Verification items for the finished model (mm, model axes). A direction names the side the tool comes from. Coordinates: 2 decimals unless noted, no trailing zeros. Order: outer loops, then holes, each group sorted by start corner. A loop starts at its lowest first (then second) coordinate and runs counter-clockwise, first axis right, second up. Notation, with made-up numbers: M 65,29 L 76,29 A34 ccw 76,66 Z; hole C 68,63.25 d2. An arc over 180 degrees is marked long. Write item = value, one per line.
```python
from build123d import *

# Parameters (mm, degrees)
F0_R     = 20
F1_DEPTH = 450
F2_R     = 35
F3_DEPTH = 24
F4_W     = 60
F4_H     = 45
F5_DEPTH = 25
F5_TAPER = -18.1


with BuildPart() as f1:
    # F0 (on Top) → F1 (new body)
    with BuildSketch(Plane.XY):
        Circle(F0_R)
    extrude(amount=F1_DEPTH)

    # F2 (on face) → F3 (join)
    with BuildSketch(Plane.XY.offset(450)):
        Circle(F2_R)
    extrude(amount=F3_DEPTH)

    # F4 (on Top) → F5 (join)
    with BuildSketch(Plane.XY):
        Rectangle(F4_W, F4_H)
    extrude(amount=-F5_DEPTH, taper=F5_TAPER)


solid = f1.part
```
Item 1: Gauge pin test, flat ends, axial feed: pin 1 (6 mm diameter, centred on y = 2, z = 206.5, fed in from -X); pin 2 (10 mm diameter, centred on x = -18.5, z = 53, fed in from +Y); pin 3 (10 mm diameter, centred on y = 22.5, z = 355.5, fed in from +X). Record the tip position at first contact, or that the pin passes through.
Report:
pin_1 = -20
pin_2 = 14.76
pin_3 = 9.68
Item 2: Scan lines: L1, parallel to Z at x = 18, y = -9.5; L2, parallel to Y at x = -4, z = 314.5; L3, parallel to Y at x = 5.5, z = 358. Record each from-to range of solid material in increasing order. Write a range as from..to.
Report:
L1 = -25..0, 450..474
L2 = -19.6..19.6
L3 = -19.23..19.23
Item 3: Sectioned sample at A-A, the plane z = 205.5. Enter the section's corners in (x, y), then the cut area to 3 significant figures.
Report:
outline = C 0,0 d40
area = 1,260 mm^2
Item 4: Tool access check on faces 5 (the flat face through (18, -10, 0)), 6 (the cylindrical face through (-28, -21, 462)). Record the directions out of +Z, -Z, +X, -X, +Y, -Y that give a thin tool (end or side, any length) a straight path to the whole face; none if there is none.
Report:
face_5 = none
face_6 = +Z
Item 5: Release check for a two-part mould opening along Z. For faces 1 (the cylindrical face through (-4.336, -19.524, 221.85)), 2 (the flat face through (0, 0, 474)), 3 (the flat face through (15, -15, 450)), 4 (the flat face through (-1, 0, -25)) record: pulls with the +Z half, pulls with the -Z half, needs draft (parallel to the pull), parting line crosses it, or undercut.
Report:
face_1 = undercut
face_2 = pulls with the +Z half
face_3 = undercut
face_4 = pulls with the -Z half
